```python
from build123d import *

# Parameters (mm, degrees)
SKETCH1_W           = 37
SKETCH1_H           = 32
BOSS_EXTRUDE1_DEPTH = 19.5
SKETCH1_3_R         = 1.5
CUT_EXTRUDE1_DEPTH  = 10
FILLET1_R           = 3


with BuildPart() as part:
    # Sketch1 → Boss-Extrude1 (new body)
    with BuildSketch(Plane(origin=(0, 0, 0), x_dir=(1, 0, 0), z_dir=(0, 1, 0))):
        Rectangle(SKETCH1_W, SKETCH1_H)
    extrude(amount=-BOSS_EXTRUDE1_DEPTH)

    # Sketch1_3 → Cut-Extrude1 (cut)
    with BuildSketch(Plane(origin=(0, 0, 0), x_dir=(1, 0, 0), z_dir=(0, 1, 0))):
        with Locations(Location((-10, 10, 0), (0, 0, 270))):
            Circle(SKETCH1_3_R)
        with Locations(Location((10, 10, 0), (0, 0, 270))):
            Circle(SKETCH1_3_R)
        with Locations(Location((10, -10, 0), (0, 0, 270))):
            Circle(SKETCH1_3_R)
        with Locations(Location((-10, -10, 0), (0, 0, 270))):
            Circle(SKETCH1_3_R)
    extrude(amount=-CUT_EXTRUDE1_DEPTH, mode=Mode.SUBTRACT)

    # Fillet1
    fillet1_edges = [part.edges().sort_by_distance(p)[0] for p in [
        (-18.5, -9.75, 16),
        (-18.5, -9.75, -16),
        (18.5, -9.75, -16),
        (18.5, -9.75, 16),
    ]]
    fillet(fillet1_edges, radius=FILLET1_R)


solid = part.part
```
The listing builds one solid part. Answer for the finished solid, in the listing's coordinates (mm). A direction names the side the tool comes from. Coordinates: 2 decimals unless noted, no trailing zeros. Loops run counter-clockwise (first coordinate to the right, second up) from the corner with the lowest first, then second, coordinate; pieces in that order, holes last. Notation, with made-up numbers: (80, 74.25) - (86, 74.25) arc R32 cw to (86, 106.25) - close; hole circle Ø8 at (73, 39). An arc over 180 degrees is marked (long way). Write item = value, one per line.
1) Section B-B (z = -10) is taken. Determine the outline of the cut face in (x, y).
Responses:
outline = (-18.5, -19.5) - (18.5, -19.5) - (18.5, 0) - (11.5, 0) - (11.5, -10) - (8.5, -10) - (8.5, 0) - (-8.5, 0) - (-8.5, -10) - (-11.5, -10) - (-11.5, 0) - (-18.5, 0) - close
2) Section A-A (y = -8.75) is taken. Determine the outline of the cut face in (x, z), plus the area to 3 significant figures.
Responses:
outline = (-18.5, -13) arc R3 ccw to (-15.5, -16) - (15.5, -16) arc R3 ccw to (18.5, -13) - (18.5, 13) arc R3 ccw to (15.5, 16) - (-15.5, 16) arc R3 ccw to (-18.5, 13) - close; hole circle Ø3 at (-10, -10); hole circle Ø3 at (-10, 10); hole circle Ø3 at (10, -10); hole circle Ø3 at (10, 10)
area = 1,150 mm^2
3) Which of the six approach directions +Z, -Z, +X, -X, +Y, -Y give full straight-line access (tool end or side, diameter ignored) to faces 4 (the face through (0, -10, 16)), 5 (the face through (9.1, -4.9, -11.2))?
Responses:
face_4 = +Z, +X, -X, +Y, -Y
face_5 = +Y
4) Determine the mould class of faces 1 (the face through (0, 0, 0)), 2 (the face through (9.1, -4.9, 8.8)), 3 (the face through (-17.64, -9.89, -15.1)) for opening direction Z: pulls with the +Z half, pulls with the -Z half, needs draft (parallel to the pull), parting line crosses it, or undercut.
Responses:
face_1 = needs draft
face_2 = undercut
face_3 = pulls with the -Z half
5) This flat-tipped pin is pushed along its axis until it touches: P1, Ø2.5, axis at x = 10, z = 10, coming from the +Y side. Where does it stop, or does it pass through?
Responses:
P1 = -10
6) Find the intervals of material crossed by line 1 along X through (y, z) = (-5.75, -10); line 2 along Z through (x, y) = (-9.5, -8.5); line 3 along X through (y, z) = (-7.5, 14.5), in increasing order.
Responses:
line_1 = -18.5 to -11.5, -8.5 to 8.5, 11.5 to 18.5
line_2 = -16 to -11.41, -8.59 to 8.59, 11.41 to 16
line_3 = -18.1 to 18.1
7) Section C-C (x = 10) is taken. Determine the outline of the cut face in (y, z), plus the area to 3 significant figures.
Responses:
outline = (-19.5, -16) - (0, -16) - (0, -11.5) - (-10, -11.5) - (-10, -8.5) - (0, -8.5) - (0, 8.5) - (-10, 8.5) - (-10, 11.5) - (0, 11.5) - (0, 16) - (-19.5, 16) - close
area = 564 mm^2
